Verification items for this drawing (mm, ordinates from the low corner). Coordinates: 2 decimals unless noted, no trailing zeros. Loops run counter-clockwise (first coordinate to the right, second up) from the corner with the lowest first, then second, coordinate; pieces in that order, holes last. Notation, with made-up numbers: (-35, 57) - (-23, 57) arc R22 cw to (-23, 70) - close; hole circle Ø2 at (27, 54.25). An arc over 180 degrees is marked (long way). One line per item, written item: value. Start each with the question number.
(1) Gauge pin test, flat end, axial feed: P1, Ø11, axis at x = 22.05, z = 57.15, coming from the -Y side. Record the tip position at first contact, or that the pin passes through.
(2) Section check C-C (z = 57.15). Record the boundary of the cut face in (x, y) (3 decimals).
(3) Section check B-B (z = 15). Record the boundary of the cut face in (x, y) (3 decimals), plus the area to 3 significant figures.
(4) Section check D-D (y = 1.15). Count the separate pieces of the cut face and the enclosed holes in it, plus the area to 3 significant figures.
(5) Section check A-A (x = 134). Record the boundary of the cut face in (y, z) (3 decimals), plus the area to 3 significant figures.
(6) Thickness scan on probe 1 along X at (y, z) = (1.8, 47) (3 decimals); probe 2 along X at (y, z) = (2, 57.15); probe 3 along X at (y, z) = (0.8, 7.5). Record the ranges inside material, lowest first. Write a range as [from, to].
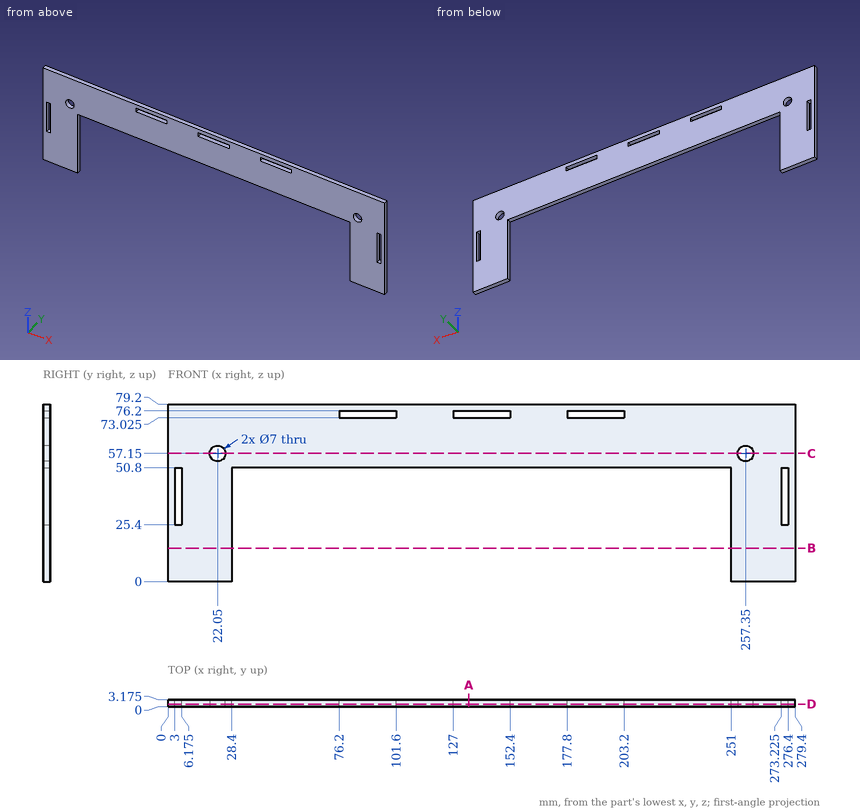
Responses:
1. P1: stops at y = 0
2. outline: (0, 0) - (18.55, 0) - (18.55, 3.175) - (0, 3.175) - close; (25.55, 0) - (253.85, 0) - (253.85, 3.175) - (25.55, 3.175) - close; (260.85, 0) - (279.4, 0) - (279.4, 3.175) - (260.85, 3.175) - close
3. outline: (0, 0) - (28.4, 0) - (28.4, 3.175) - (0, 3.175) - close; (251, 0) - (279.4, 0) - (279.4, 3.175) - (251, 3.175) - close
3. area: 180 mm²
4. separate pieces: 1
4. enclosed holes: 7
4. area: 10,300 mm²
5. outline: (0, 50.8) - (3.175, 50.8) - (3.175, 73.025) - (0, 73.025) - close; (0, 76.2) - (3.175, 76.2) - (3.175, 79.2) - (0, 79.2) - close
5. area: 80.1 mm²
6. probe 1: x = [0, 3], [6.175, 28.4], [251, 273.225], [276.4, 279.4]
6. probe 2: x = [0, 18.55], [25.55, 253.85], [260.85, 279.4]
6. probe 3: x = [0, 28.4], [251, 279.4]
